For this review, take the finished solid that the model builds, in its own axes (mm). A direction names the side the tool comes from. Coordinates: 2 decimals unless noted, no trailing zeros. Loops run counter-clockwise (first coordinate to the right, second up) from the corner with the lowest first, then second, coordinate; pieces in that order, holes last. Notation, with made-up numbers: M 17,-34 L 53,-34 A12 cw 53,-26 Z; hole C 42,61 d8. An arc over 180 degrees is marked long. Put each result on its own line as item: value.
```python
from build123d import *

# Parameters (mm, degrees)
SKETCH1_R           = 13
SKETCH1_R_2         = 3.5
SKETCH1_R_3         = 1.5
BOSS_EXTRUDE1_DEPTH = 7
SKETCH2_R           = 4.05
CUT_EXTRUDE1_DEPTH  = 5
FILLET1_R           = 3


with BuildPart() as part:
    # Sketch1 → Boss-Extrude1 (new body)
    with BuildSketch(Plane(origin=(0, 0, 0), x_dir=(1, 0, 0), z_dir=(0, 1, 0))):
        with Locations(Location((0, 0, 0), (0, 0, 270))):
            Circle(SKETCH1_R)
        with Locations(Location((0, 0, 0), (0, 0, 270))):
            Circle(SKETCH1_R_2, mode=Mode.SUBTRACT)
        with Locations(Location((0, 7, 0), (0, 0, 270))):
            Circle(SKETCH1_R_3, mode=Mode.SUBTRACT)
        with Locations(Location((7, 0, 0), (0, 0, 270))):
            Circle(SKETCH1_R_3, mode=Mode.SUBTRACT)
        with Locations(Location((0, -7, 0), (0, 0, 270))):
            Circle(SKETCH1_R_3, mode=Mode.SUBTRACT)
        with Locations(Location((-7, 0, 0), (0, 0, 270))):
            Circle(SKETCH1_R_3, mode=Mode.SUBTRACT)
    extrude(amount=BOSS_EXTRUDE1_DEPTH)

    # Sketch2 → Cut-Extrude1 (cut)
    with BuildSketch(Plane(origin=(0, 7, 0), x_dir=(1, 0, 0), z_dir=(0, 1, 0))):
        with Locations(Location((0, 0, 0), (0, 0, 270))):
            Circle(SKETCH2_R)
    extrude(amount=-CUT_EXTRUDE1_DEPTH, mode=Mode.SUBTRACT)

    # Fillet1
    fillet1_edges = [part.edges().sort_by_distance(p)[0] for p in [
        (0, 7, -13),
    ]]
    fillet(fillet1_edges, radius=FILLET1_R)


solid = part.part
```
(1) Add section B-B (x = 0). Write out the cut boundary in (y, z), plus the area to 3 significant figures.
Determined:
outline: M 0,-13 L 4,-13 A3 ccw 7,-10 L 7,-8.5 L 0,-8.5 Z; M 0,-5.5 L 7,-5.5 L 7,-4.05 L 2,-4.05 L 2,-3.5 L 0,-3.5 Z; M 0,3.5 L 2,3.5 L 2,4.05 L 7,4.05 L 7,5.5 L 0,5.5 Z; M 0,8.5 L 7,8.5 L 7,10 A3 ccw 4,13 L 0,13 Z
area: 81.6 mm^2
(2) Tool access review of faces 1 (the cylindrical face through (-3.593, 4.535, 1.869)), 2 (the cylindrical face through (-3.417, 0.986, -0.759)): name each direction out of +Z, -Z, +X, -X, +Y, -Y from which nothing blocks a thin tool from reaching the whole face with its end or side.
Determined:
face 1: +Y
face 2: +Y, -Y
(3) Add section A-A (z = 0). Write out the cut boundary in (x, y).
Determined:
outline: M -13,0 L -8.5,0 L -8.5,7 L -10,7 A3 ccw -13,4 Z; M -5.5,0 L -3.5,0 L -3.5,2 L -4.05,2 L -4.05,7 L -5.5,7 Z; M 3.5,0 L 5.5,0 L 5.5,7 L 4.05,7 L 4.05,2 L 3.5,2 Z; M 8.5,0 L 13,0 L 13,4 A3 ccw 10,7 L 8.5,7 Z
(4) Wall thickness on line 1 along X through (y, z) = (0.4, 0); line 2 along X through (y, z) = (5.5, 0); line 3 along X through (y, z) = (5.75, 8.25): over which ranges is each line inside the solid? List them lowest first. Write a range as [from, to].
Determined:
line 1: x = [-13, -8.5], [-5.5, -3.5], [3.5, 5.5], [8.5, 13]
line 2: x = [-12.6, -8.5], [-5.5, -4.05], [4.05, 5.5], [8.5, 12.6]
line 3: x = [-9.31, -0.83], [0.83, 9.31]
(5) Draft analysis for pull direction X (two halves, no side actions). For faces 3 (the flat face through (-3, 0, 3)), 4 (the cylindrical face through (0.07, 3.45, 5.5)), 5 (the cylindrical face through (-7.91, 1.972, -10.316)), state which applies: +X half, -X half, draft (parallel to the pull), parting line (faces both ways), or undercut.
Determined:
face 3: draft
face 4: undercut
face 5: parting line
(6) For pin 1 (1.5 mm diameter, centred on x = 5, z = 7.5, fed in from -Y); pin 2 (1.5 mm diameter, centred on x = -6.5, y = 1.5, fed in from +Z); pin 3 (6.5 mm diameter, centred on x = 0.5, z = 0.5, fed in from +Y); pin 4 (2.5 mm diameter, centred on x = 7, z = 0, fed in from -Y), all flat-tipped, find the tip position at first contact; note any pin that passes through.
Determined:
pin 1: stops at y = 0
pin 2: stops at z = 11.66
pin 3: stops at y = 2
pin 4: passes through
